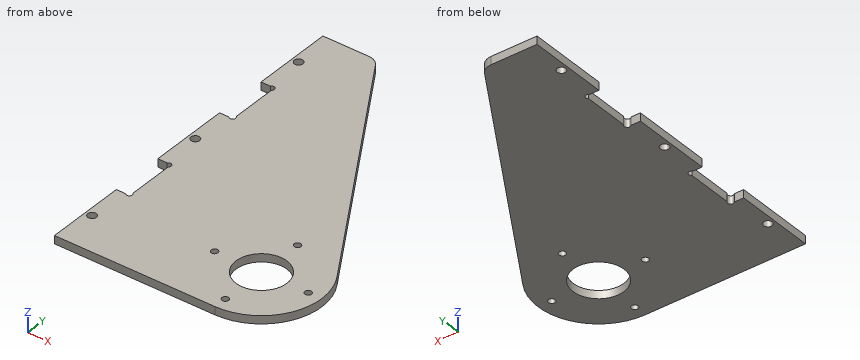
from build123d import *

# Parameters (mm, degrees)
SKETCH_2_R          = 9.5
SKETCH_2_R_2        = 1.25
EXTRUDE_1_DEPTH     = 3
FILLET_3_R          = 5
SKETCH_4_R          = 1.6
SKETCH_4_R_2        = 1.1
SKETCH_4_W          = 5.05
SKETCH_4_H          = 20.1
CUT_EXTRUDE_1_DEPTH = 10


with BuildPart() as part:
    # ｽｹｯﾁ2 → ﾎﾞｽ - 押し出し1 (new body)
    with BuildSketch(Plane.XY):
        with BuildLine():
            Line((-60, 107.5), (-60, -22.5))
            Line((-60, -22.5), (-40, -22.5))
            Line((-40, -22.5), (0, -22.5))
            ThreePointArc((0, -22.5), (19.65247344, -10.9558335), (19.138597944, 11.830641096))
            Line((19.138597944, 11.830641096), (-40, 107.5))
            Line((-40, 107.5), (-60, 107.5))
        make_face()
        Circle(SKETCH_2_R, mode=Mode.SUBTRACT)
        with Locations((0, 17.5)):
            Circle(SKETCH_2_R_2, mode=Mode.SUBTRACT)
        with Locations((17.5, 0)):
            Circle(SKETCH_2_R_2, mode=Mode.SUBTRACT)
        with Locations((0, -17.5)):
            Circle(SKETCH_2_R_2, mode=Mode.SUBTRACT)
        with Locations((-17.5, 0)):
            Circle(SKETCH_2_R_2, mode=Mode.SUBTRACT)
    extrude(amount=EXTRUDE_1_DEPTH)

    # ﾌｨﾚｯﾄ3
    fillet_3_edges = [part.edges().sort_by_distance(p)[0] for p in [
        (-40, 107.5, 1.5),
    ]]
    fillet(fillet_3_edges, radius=FILLET_3_R)

    # ｽｹｯﾁ4 → ｶｯﾄ - 押し出し1 (cut)
    with BuildSketch(Plane.XY.offset(3)):
        with Locations((-57.5, -7.5)):
            Circle(SKETCH_4_R)
        with Locations((-57.5, 42.5)):
            Circle(SKETCH_4_R)
        with Locations((-57.5, 92.5)):
            Circle(SKETCH_4_R)
        with Locations((-55.61, 26.89)):
            Circle(SKETCH_4_R_2)
        with Locations((-55.61, 8.11)):
            Circle(SKETCH_4_R_2)
        with Locations((-55.61, 58.11)):
            Circle(SKETCH_4_R_2)
        with Locations((-55.61, 76.89)):
            Circle(SKETCH_4_R_2)
        with Locations((-57.475, 67.5)):
            Rectangle(SKETCH_4_W, SKETCH_4_H)
        with Locations((-57.475, 17.5)):
            Rectangle(SKETCH_4_W, SKETCH_4_H)
    extrude(amount=-CUT_EXTRUDE_1_DEPTH, mode=Mode.SUBTRACT)


solid = part.part
The listing builds one solid part. Answer for the finished solid, in the listing's coordinates (mm). Round coordinates to 2 decimals unless told otherwise and drop trailing zeros. Order: outer loops, then holes, each group sorted by start corner. A loop starts at its lowest first (then second) coordinate and runs counter-clockwise, first axis right, second up. Notation, with made-up numbers: M 18,63.25 L 23,63.25 A11 ccw 23,83.25 Z; hole C 17.5,-14 d9. An arc over 180 degrees is marked long. Answer in a Markdown table with one row per item. Add a question column.
1) A flat-ended cylindrical pin translates along its axis: pin 1 Ø1.8 at (x, y) = (-55.61, 8.11) entering from +Z. Find the tip coordinate at first contact, or state that the pin passes through.
2) Consider line 1 along Y through (x, z) = (-57.5, 1.15); line 2 along Y through (x, z) = (-55.61, 2.25); line 3 along X through (y, z) = (43, 2.6). Determine where each line is inside the solid, lowest interval first. Write a range as from..to.
3) The part is cut by section B-B on z = 0.45. Count the separate pieces of the cut face and the enclosed holes in it, plus the area to 3 significant figures.
4) The part is cut by section C-C on x = 17.5. Determine the outline of the cut face in (y, z).
5) The part is cut by section A-A on y = 0. Determine the outline of the cut face in (x, z), plus the area to 4 significant figures.
6) The part is cut by section D-D on y = 17.5. Determine the outline of the cut face in (x, z).
Findings below:
| question | item | result |
|---|---|---|
| 1 | pin 1 | passes through |
| 2 | line 1 | y = -22.5..-9.1, -5.9..7.45, 27.55..40.9, 44.1..57.45, 77.55..90.9, 94.1..107.5 |
| 2 | line 2 | y = -22.5..7.01, 27.99..57.01, 77.99..107.5 |
| 2 | line 3 | x = -60..-59.02, -55.98..-0.13 |
| 3 | separate pieces | 1 |
| 3 | enclosed holes | 8 |
| 3 | area | 6,920 mm² |
| 4 | outline | M -14.14,0 L -1.25,0 L -1.25,3 L -14.14,3 Z; M 1.25,0 L 14.48,0 L 14.48,3 L 1.25,3 Z |
| 5 | outline | M -60,0 L -18.75,0 L -18.75,3 L -60,3 Z; M -16.25,0 L -9.5,0 L -9.5,3 L -16.25,3 Z; M 9.5,0 L 16.25,0 L 16.25,3 L 9.5,3 Z; M 18.75,0 L 22.5,0 L 22.5,3 L 18.75,3 Z |
| 5 | area | 175.5 mm² |
| 6 | outline | M -54.95,0 L -1.25,0 L -1.25,3 L -54.95,3 Z; M 1.25,0 L 15.63,0 L 15.63,3 L 1.25,3 Z |
